Here's how the part is built. I have some questions about the finished solid (model axes, mm). A direction names the side the tool comes from. Round coordinates to 2 decimals unless told otherwise and drop trailing zeros. Order: outer loops, then holes, each group sorted by start corner. A loop starts at its lowest first (then second) coordinate and runs counter-clockwise, first axis right, second up.
```python
from build123d import *

# Parameters (mm, degrees)
SKETCH1_R               = 6
BOSS_EXTRUDE1_DEPTH     = 5
BOSS_EXTRUDE2_START     = -5
BOSS_EXTRUDE2_DEPTH     = 5
CUT_EXTRUDE1_DEPTH      = 5
SKETCH4_R               = 15
BOSS_EXTRUDE3_DEPTH     = 15
SKETCH5_R               = 15
BOSS_EXTRUDE4_DEPTH     = 2
SKETCH6_R               = 15
SKETCH6_W               = 16
SKETCH6_H               = 16
BOSS_EXTRUDE5_DEPTH     = 15
CUT_EXTRUDE2_DEPTH      = 51
CUT_EXTRUDE5_DEPTH      = 1
CUT_EXTRUDE5_DEPTH_BACK = 51
SKETCH10_R              = 2.6
CUT_EXTRUDE6_DEPTH      = 7


with BuildPart() as part:
    # Sketch1 → Boss-Extrude1 (new body)
    with BuildSketch(Plane(origin=(0, 0, 0), x_dir=(1, 0, 0), z_dir=(0, 1, 0))):
        with Locations(Location((0, 0, 0), (0, 0, 270))):
            Circle(SKETCH1_R)
        with BuildLine():
            ThreePointArc((-1.549193338, 2.15), (0, -2.65), (1.549193338, 2.15))
            Line((1.549193338, 2.15), (-1.549193338, 2.15))
        make_face(mode=Mode.SUBTRACT)
    extrude(amount=BOSS_EXTRUDE1_DEPTH)

    # Sketch2 → Boss-Extrude2 (add)
    with BuildSketch(Plane(origin=(0, 5, 0), x_dir=(1, 0, 0), z_dir=(0, 1, 0)).offset(BOSS_EXTRUDE2_START)):
        with BuildLine():
            Line((1.549193338, 2.15), (-1.549193338, 2.15))
            ThreePointArc((-1.549193338, 2.15), (0, -2.65), (1.549193338, 2.15))
        make_face()
        with BuildLine():
            Line((1.526433752, 2.08), (-1.526433752, 2.08))
            ThreePointArc((-1.526433752, 2.08), (0, -2.58), (1.526433752, 2.08))
        make_face(mode=Mode.SUBTRACT)
    extrude(amount=BOSS_EXTRUDE2_DEPTH)

    # Sketch3 → Cut-Extrude1 (cut)
    with BuildSketch(Plane(origin=(0, 5, 0), x_dir=(1, 0, 0), z_dir=(0, 1, 0))):
        with BuildLine():
            Line((1.532970972, 2.1), (-1.532970972, 2.1))
            ThreePointArc((-1.532970972, 2.1), (0, -2.6), (1.532970972, 2.1))
        make_face()
    extrude(amount=-CUT_EXTRUDE1_DEPTH, mode=Mode.SUBTRACT)

    # Sketch4 → Boss-Extrude3 (add)
    with BuildSketch(Plane(origin=(0, 5, 0), x_dir=(1, 0, 0), z_dir=(0, 1, 0))):
        with Locations(Location((0, 0, 0), (0, 0, 270))):
            Circle(SKETCH4_R)
        with BuildLine():
            Line((1.532970972, 2.1), (-1.532970972, 2.1))
            ThreePointArc((-1.532970972, 2.1), (0, -2.6), (1.532970972, 2.1))
        make_face(mode=Mode.SUBTRACT)
    extrude(amount=-BOSS_EXTRUDE3_DEPTH)

    # Sketch5 → Boss-Extrude4 (add)
    with BuildSketch(Plane.XZ.offset(10)):
        with Locations(Location((0, 0, 0), (0, 0, 90))):
            Circle(SKETCH5_R)
    extrude(amount=BOSS_EXTRUDE4_DEPTH)

    # Sketch6 → Boss-Extrude5 (add)
    with BuildSketch(Plane.XZ.offset(12)):
        with Locations(Location((0, 0, 0), (0, 0, 90))):
            Circle(SKETCH6_R)
        Rectangle(SKETCH6_W, SKETCH6_H, mode=Mode.SUBTRACT)
    extrude(amount=BOSS_EXTRUDE5_DEPTH)

    # Sketch7 → Cut-Extrude2 (cut)
    with BuildSketch(Plane(origin=(0, 5, 0), x_dir=(1, 0, 0), z_dir=(0, 1, 0))):
        with BuildLine():
            Line((0, 14), (0, 15))
            ThreePointArc((0, 15), (-2.738612788, 14.747881204), (-5.385164807, 14))
            Line((-5.385164807, 14), (0, 14))
        make_face()
        with BuildLine():
            ThreePointArc((5.385164807, 14), (2.738612788, 14.747881204), (0, 15))
            Line((0, 15), (0, 14))
            Line((0, 14), (5.385164807, 14))
        make_face()
    extrude(amount=-CUT_EXTRUDE2_DEPTH, mode=Mode.SUBTRACT)

    # Sketch8 → Cut-Extrude5 (cut, two sides: drawn at the far end of the back side and taken through both)
    with BuildSketch(Plane.XY.offset(-2.1).offset(-CUT_EXTRUDE5_DEPTH_BACK)):
        with BuildLine():
            Line((1.532970972, -2.041742431), (1.532970972, -2.5))
            Line((1.532970972, -2.5), (1.532970972, -2.958257569))
            ThreePointArc((1.532970972, -2.958257569), (1.58315406, -2.731566886), (1.6, -2.5))
            ThreePointArc((1.6, -2.5), (1.58315406, -2.268433114), (1.532970972, -2.041742431))
        make_face()
        with BuildLine():
            Line((-1.532970972, -2.041742431), (-1.532970972, -2.5))
            Line((-1.532970972, -2.5), (1.532970972, -2.5))
            Line((1.532970972, -2.5), (1.532970972, -2.041742431))
            ThreePointArc((1.532970972, -2.041742431), (0, -0.9), (-1.532970972, -2.041742431))
        make_face()
        with BuildLine():
            Line((1.532970972, -2.5), (-1.532970972, -2.5))
            Line((-1.532970972, -2.5), (-1.532970972, -2.958257569))
            ThreePointArc((-1.532970972, -2.958257569), (0, -4.1), (1.532970972, -2.958257569))
            Line((1.532970972, -2.958257569), (1.532970972, -2.5))
        make_face()
        with BuildLine():
            Line((-1.532970972, -2.958257569), (-1.532970972, -2.5))
            Line((-1.532970972, -2.5), (-1.532970972, -2.041742431))
            ThreePointArc((-1.532970972, -2.041742431), (-1.6, -2.5), (-1.532970972, -2.958257569))
        make_face()
    extrude(amount=CUT_EXTRUDE5_DEPTH + CUT_EXTRUDE5_DEPTH_BACK, mode=Mode.SUBTRACT)

    # Sketch10 → Cut-Extrude6 (cut)
    with BuildSketch(Plane(origin=(0, 0, -14), x_dir=(-1, 0, 0), z_dir=(0, 0, -1))):
        with Locations((0, -2.5)):
            Circle(SKETCH10_R)
    extrude(amount=-CUT_EXTRUDE6_DEPTH, mode=Mode.SUBTRACT)


solid = part.part
```
1. On a 3-axis mill with a long thin cutter (end or side, diameter ignored), from which of +Z, -Z, +X, -X, +Y, -Y can I reach the whole of each face in a straight line? I mean faces 1 (the flat face through (0, -27, -9)), 2 (the flat face through (-1, -1, -7)), 3 (the flat face through (0, -10, 0)), 4 (the flat face through (8, -19, 0)), 5 (the flat face through (0, 5, -3)). Say none if no direction works.
Evaluation:
face 1: +Z, -Z, +X, -X, -Y
face 2: -Z
face 3: +Y
face 4: -Y
face 5: +Z, -Z, +X, -X, +Y
2. If we section it at A-A, the plane x = 0: Write out the boundary of the cut face in (y, z).
Evaluation:
outline: (-27, -14) - (-5.1, -14) - (-5.1, -7) - (-4.1, -7) - (-4.1, -2.1) - (-10, -2.1) - (-10, 2.6) - (5, 2.6) - (5, 15) - (-27, 15) - (-27, 8) - (-12, 8) - (-12, -8) - (-27, -8) - close; (-0.9, -7) - (0.1, -7) - (0.1, -14) - (5, -14) - (5, -2.1) - (-0.9, -2.1) - close
3. If we section it at C-C, the plane y = -16.5: Write out the boundary of the cut face in (x, z).
Evaluation:
outline: (-5.39, -14) - (5.39, -14) arc R15 ccw (long way) to start; hole (-8, -8) - (8, -8) - (8, 8) - (-8, 8) - close
4. If we mould it in two halves opening along X, with no side actions, what happens to faces 6 (the flat face through (0, -11, -14)), 7 (the cylindrical face through (-1.2, -4.807, -10.549)), 8 (the cylindrical face through (0.58, -10.78, 14.99))? For each: released by +X, released by -X, zero draft, split by the parting line, or undercut.
Evaluation:
face 6: zero draft
face 7: undercut
face 8: split by the parting line
5. I'm going to push flat-ended pins straight in: P1, Ø4, axis at x = 4, z = -2, coming from the -Y side; P2, Ø6, axis at y = -23, z = 7.5, coming from the +X side; P3, Ø10, axis at y = -4.5, z = 7, coming from the -X side. Where does each tip first touch, or does it pass through?
Evaluation:
P1: stops at y = -12
P2: stops at x = 14.31
P3: stops at x = -14.87
6. If we section it at D-D, the plane x = -12: Write out the boundary of the cut face in (y, z).
Evaluation:
outline: (-27, -9) - (5, -9) - (5, 9) - (-27, 9) - close
7. I need wall thicknesses on probe 1 along Y at (x, z) = (0, -8.25); probe 2 along Z at (x, y) = (0, -4.75); probe 3 along Y at (x, z) = (-2.5, 6.5). Which ranges of each line are inside material? Lowest first, please.
Evaluation:
probe 1: y = -27 to -5.1, 0.1 to 5
probe 2: z = -7 to -2.1, 2.6 to 15
probe 3: y = -12 to 5
8. If we section it at B-B, the plane z = 0: Write out the boundary of the cut face in (x, y), and give its area (3 significant figures).
Evaluation:
outline: (-15, -27) - (-8, -27) - (-8, -12) - (8, -12) - (8, -27) - (15, -27) - (15, 5) - (2.6, 5) - (2.6, -10) - (-2.6, -10) - (-2.6, 5) - (-15, 5) - close
area: 642 mm2
